Check sheet for the modelled part. Datum: model origin and axes. Units: mm. Round coordinates to 2 decimals unless told otherwise and drop trailing zeros. Loops run counter-clockwise (first coordinate to the right, second up) from the corner with the lowest first, then second, coordinate; pieces in that order, holes last. Notation, with made-up numbers: (52, 41) -> (95, 41) arc R21 ccw to (95, 61) -> close; hole circle Ø2 at (52.5, 79.5). An arc over 180 degrees is marked (long way). Use one line per item in the form item = value. Start each with the question number.
(1) Sectioned sample at D-D (x = -28). Record the cut outline in (y, z) (3 decimals).
(2) Go/stop test with flat-tipped pins: pin 1 (15 mm diameter, centred on x = -124, y = 38, fed in from +Z); pin 2 (6 mm diameter, centred on y = 29, z = -19, fed in from -X); pin 3 (15 mm diameter, centred on x = -50, y = 24.5, fed in from -Z). Record where each tip stops, or that it passes through.
(3) Sectioned sample at B-B (x = 26). Record the cut outline in (y, z) (3 decimals).
(4) Material ranges on probe 1 along X at (y, z) = (30, 130); probe 2 along X at (y, z) = (25, 140); probe 3 along Z at (x, y) = (-105.5, 35.5), recorded low to high. Write a range as [from, to].
(5) Draft check along Z on faces 1 (the cylindrical face through (149.922, 26.547, 95.584)), 2 (the flat face through (-44.05, 28.22, 78.84)), 3 (the flat face through (-118, 53.848, 131)), 4 (the cylindrical face through (1.26, 28.87, -174.62)). Enter one of: released by +Z, released by -Z, zero draft, split by the parting line, or undercut.
(6) Sectioned sample at C-C (z = 35.5). Record the cut outline in (x, y) (3 decimals), and give its area (3 significant figures).
(7) Sectioned sample at A-A (y = 25). Record the cut outline in (x, z) (3 decimals), and give its area (3 significant figures).
from build123d import *

# Parameters (mm, degrees)
SKETCH1_R           = 177.8
BOSS_EXTRUDE1_DEPTH = 53.848
SKETCH2_R           = 174.625
CUT_EXTRUDE1_DEPTH  = 50.673
SKETCH3_W           = 351.952724098
SKETCH3_H           = 2.54
EXTRUDE_THIN1_DEPTH = 50.8


with BuildPart() as part:
    # Sketch1 → Boss-Extrude1 (new body)
    with BuildSketch(Plane(origin=(0, 0, 0), x_dir=(1, 0, 0), z_dir=(0, 1, 0))):
        with Locations(Location((0, 0, 0), (0, 0, 270))):
            Circle(SKETCH1_R)
    extrude(amount=BOSS_EXTRUDE1_DEPTH)

    # Sketch2 → Cut-Extrude1 (cut)
    with BuildSketch(Plane(origin=(0, 53.848, 0), x_dir=(1, 0, 0), z_dir=(0, 1, 0))):
        with Locations(Location((0, 0, 0), (0, 0, 270))):
            Circle(SKETCH2_R)
    extrude(amount=-CUT_EXTRUDE1_DEPTH, mode=Mode.SUBTRACT)

    # Sketch3 → Extrude-Thin1 (add)
    with BuildSketch(Plane(origin=(0, 3.175, 0), x_dir=(1, 0, 0), z_dir=(0, 1, 0))):
        Polygon((86.888328762, 153.035), (-89.088033287, -151.765), (-86.888328762, -153.035), (89.088033287, 151.765), align=None)
        Polygon((-89.088033287, 151.765), (86.888328762, -153.035), (89.088033287, -151.765), (-86.888328762, 153.035), align=None)
        Rectangle(SKETCH3_W, SKETCH3_H)
    extrude(amount=EXTRUDE_THIN1_DEPTH)


solid = part.part
Checks:
q1.outline = (0, -175.581) -> (53.848, -175.581) -> (53.848, -172.366) -> (3.175, -172.366) -> (3.175, -51.037) -> (53.975, -51.037) -> (53.975, -45.957) -> (3.175, -45.957) -> (3.175, -1.27) -> (53.975, -1.27) -> (53.975, 1.27) -> (3.175, 1.27) -> (3.175, 45.957) -> (53.975, 45.957) -> (53.975, 51.037) -> (3.175, 51.037) -> (3.175, 172.366) -> (53.848, 172.366) -> (53.848, 175.581) -> (0, 175.581) -> close
q2.pin_1 = 134.32
q2.pin_2 = -177.08
q2.pin_3 = -172.65
q3.outline = (0, -175.889) -> (53.848, -175.889) -> (53.848, -172.679) -> (3.175, -172.679) -> (3.175, -47.573) -> (53.975, -47.573) -> (53.975, -42.493) -> (3.175, -42.493) -> (3.175, -1.27) -> (53.975, -1.27) -> (53.975, 1.27) -> (3.175, 1.27) -> (3.175, 42.493) -> (53.975, 42.493) -> (53.975, 47.573) -> (3.175, 47.573) -> (3.175, 172.679) -> (53.848, 172.679) -> (53.848, 175.889) -> (0, 175.889) -> close
q4.probe_1 = [-121.3, -116.59], [-76.52, -73.59], [73.59, 76.52], [116.59, 121.3]
q4.probe_2 = [-109.6, -104.37], [-82.3, -79.36], [79.36, 82.3], [104.37, 109.6]
q4.probe_3 = [-143.12, -139.15], [-1.27, 1.27], [139.15, 143.12]
q5.face_1 = split by the parting line
q5.face_2 = undercut
q5.face_3 = zero draft
q5.face_4 = undercut
q6.outline = (-174.22, 0) -> (174.22, 0) -> (174.22, 53.848) -> (170.978, 53.848) -> (170.978, 3.175) -> (21.962, 3.175) -> (21.962, 53.975) -> (19.029, 53.975) -> (19.029, 3.175) -> (-19.029, 3.175) -> (-19.029, 53.975) -> (-21.962, 53.975) -> (-21.962, 3.175) -> (-170.978, 3.175) -> (-170.978, 53.848) -> (-174.22, 53.848) -> close
q6.area = 1,730 mm2
q7.outline = circle Ø355.6 at (0, 0); hole (-174.62, -1.27) arc R174.625 ccw to (-88.41, -150.591) -> (-2.2, -1.27) -> close; hole (-174.62, 1.27) -> (-2.2, 1.27) -> (-88.41, 150.591) arc R174.625 ccw to start; hole (-86.21, -151.861) arc R174.625 ccw to (86.21, -151.861) -> (0, -2.54) -> close; hole (-86.21, 151.861) -> (0, 2.54) -> (86.21, 151.861) arc R174.625 ccw to start; hole (2.2, -1.27) -> (88.41, -150.591) arc R174.625 ccw to (174.62, -1.27) -> close; hole (2.2, 1.27) -> (174.62, 1.27) arc R174.625 ccw to (88.41, 150.591) -> close
q7.area = 6,160 mm2
